Part print with two shaded views. Sizes in mm from the minimum x, y, z corner. A direction names the side the tool comes from. Round coordinates to 2 decimals unless told otherwise and drop trailing zeros. Loops run counter-clockwise (first coordinate to the right, second up) from the corner with the lowest first, then second, coordinate; pieces in that order, holes last.
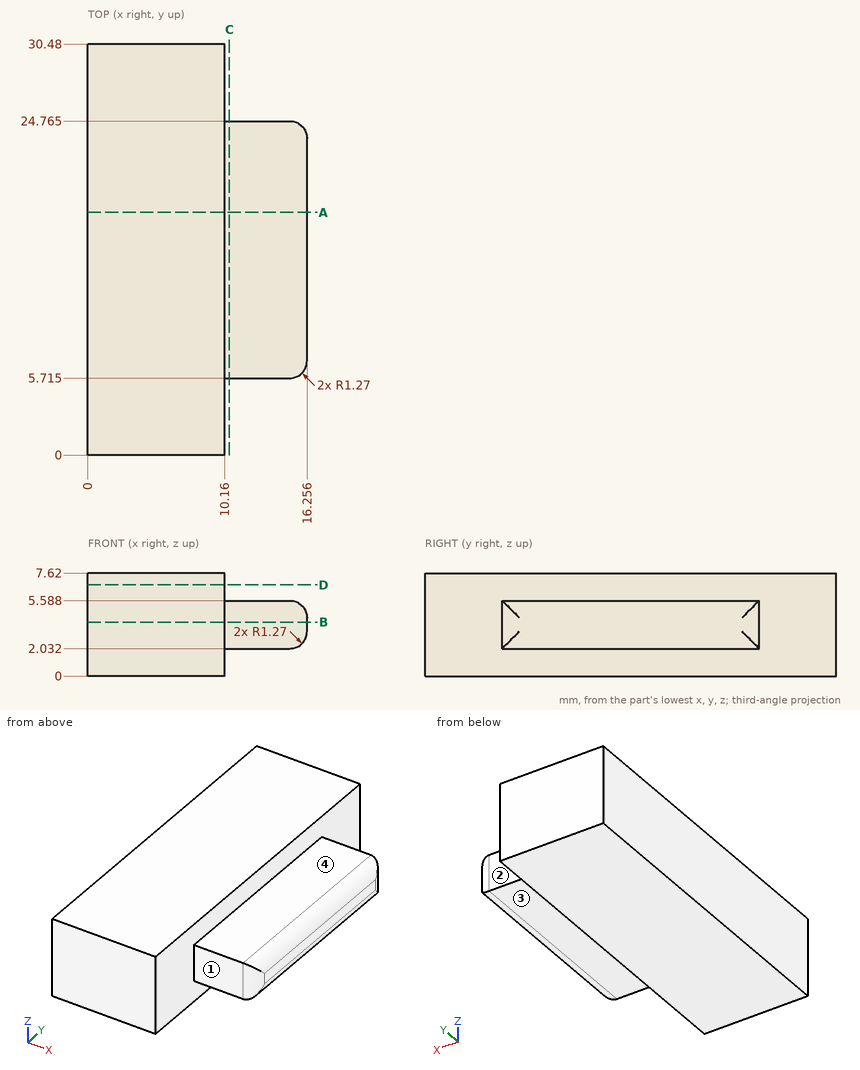
Item 1: Cut at C-C (x = 10.5). List the corners of the cut face in (y, z) (3 decimals), plus the area to 3 significant figures.
Verdict:
outline: (5.715, 2.032) - (24.765, 2.032) - (24.765, 5.588) - (5.715, 5.588) - close
area: 67.7 mm2
Item 2: Wall check: L1, parallel to Z at x = 11, y = 12; L2, parallel to X at y = 28, z = 6.75; L3, parallel to Y at x = 11.5, z = 3.75 (3 decimals). Give the ranges that are in metal, low to high.
Verdict:
L1: z = 2.03 to 5.59
L2: x = 0 to 10.16
L3: y = 5.715 to 24.765
Item 3: Cut at B-B (z = 4). List the corners of the cut face in (x, y) (3 decimals), plus the area to 3 significant figures.
Verdict:
outline: (0, 0) - (10.16, 0) - (10.16, 5.715) - (14.986, 5.715) arc R1.27 ccw to (16.256, 6.985) - (16.256, 23.495) arc R1.27 ccw to (14.986, 24.765) - (10.16, 24.765) - (10.16, 30.48) - (0, 30.48) - close
area: 425 mm2
Item 4: Cut at A-A (y = 18). List the corners of the cut face in (x, z), plus the area to 3 significant figures.
Verdict:
outline: (0, 0) - (10.16, 0) - (10.16, 2.03) - (14.99, 2.03) arc R1.27 ccw to (16.26, 3.3) - (16.26, 4.32) arc R1.27 ccw to (14.99, 5.59) - (10.16, 5.59) - (10.16, 7.62) - (0, 7.62) - close
area: 98.4 mm2
Item 5: 3-axis set-ups, long thin cutter, end or side, ignore diameter. For the marked faces 1, 2, 3 and 4: which of +Z, -Z, +X, -X, +Y, -Y reach the whole face in a straight line?
Verdict:
face 1: +Z, -Z, +X, -Y
face 2: +Z, -Z, +X, +Y
face 3: -Z, +X, +Y, -Y
face 4: +Z, +X, +Y, -Y
Item 6: Flat gauge pins, fed straight in: P1, Ø1.4, axis at x = 13.5, y = 17.5, coming from the -Z side; P2, Ø1.1, axis at x = 13.5, z = 3.5, coming from the -Y side (3 decimals); P3, Ø1.5, axis at x = 4, z = 1, coming from the -Y side; P4, Ø1.4, axis at x = 11.5, y = 19.5, coming from the +Z side. Where does each tip first touch, or does it go through?
Verdict:
P1: stops at z = 2.03
P2: stops at y = 5.715
P3: stops at y = 0
P4: stops at z = 5.59
Item 7: Cut at D-D (z = 6.75). List the corners of the cut face in (x, y), plus the area to 3 significant figures.
Verdict:
outline: (0, 0) - (10.16, 0) - (10.16, 30.48) - (0, 30.48) - close
area: 310 mm2
